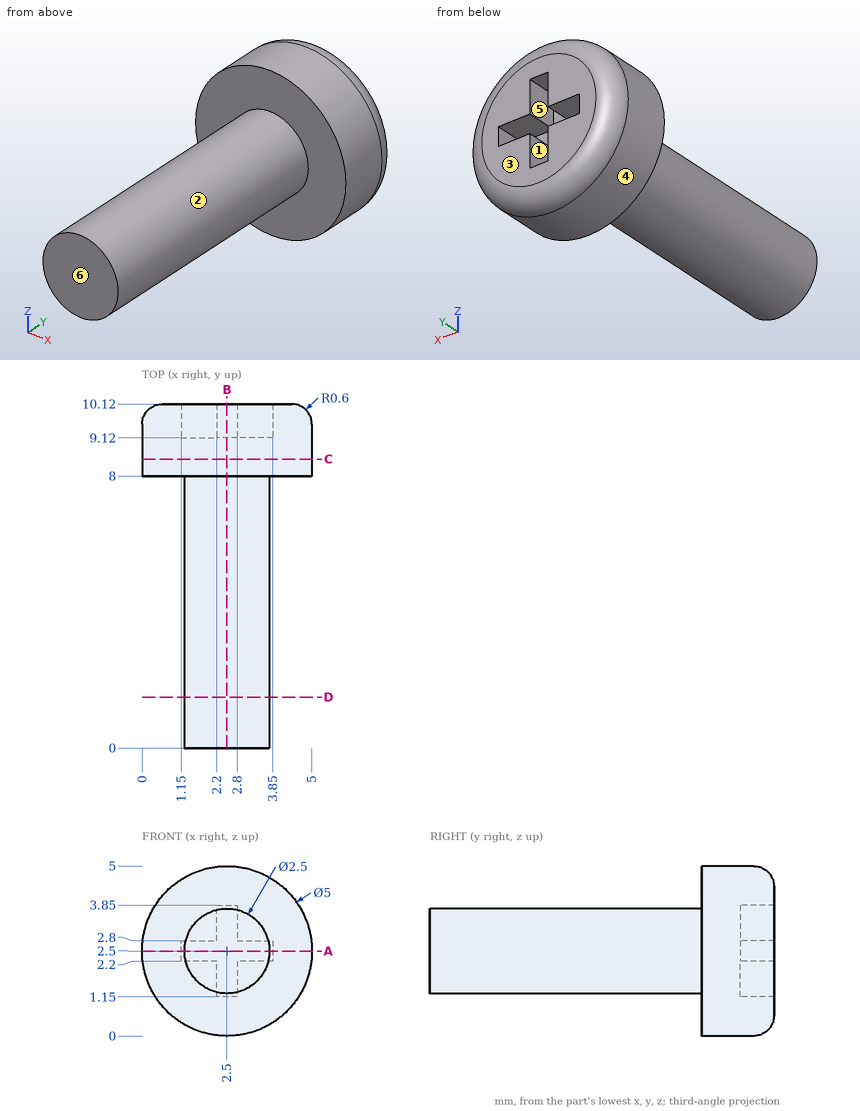
Study the drawing (mm; zero at the part's minimum x, y, z) and answer. A direction names the side the tool comes from. Coordinates: 2 decimals unless noted, no trailing zeros. Write each loop counter-clockwise with the first axis right and the second up, starting at its lowest first coordinate (ties: lowest second). Pieces come first, ordered by that corner, then holes. Notation, with made-up numbers: (-26.75, 11.25) - (-7.75, 11.25) arc R17 ccw to (-7.75, 38.25) - close; hole circle Ø6 at (-4, 67.25). An arc over 180 degrees is marked (long way). Answer as a JSON object with one key per item and string values. Group by question number.
1. Which of the six approach directions +Z, -Z, +X, -X, +Y, -Y give full straight-line access (tool end or side, diameter ignored) to the marked faces 1, 2 and 3?
2. Each of these flat-tipped pins is pushed along its axis until it touches: P1, Ø0.8, axis at x = 3.5, y = 9.5, coming from the -Z side; P2, Ø1, axis at y = 1.5, z = 0.5, coming from the -X side; P3, Ø1.5, axis at x = 3, z = 4.5, coming from the -Y side; P4, Ø1.5, axis at y = 1, z = 1, coming from the -X side. Where does it stop, or does it pass through?
3. A cutting plane is placed at C-C (y = 8.5). Determine the outline of the cut face in (x, z).
4. A cutting plane is placed at B-B (x = 2.5). Determine the outline of the cut face in (y, z), plus the area to 3 significant figures.
5. Consider L1, parallel to Y at x = 4.2, z = 2.9; L2, parallel to Y at x = 2.45, z = 2.2; L3, parallel to Z at x = 2.7, y = 8.5. Determine where each line is inside the solid, lowest interval first. Write a range as [from, to].
6. A cutting plane is placed at D-D (y = 1.5). Determine the outline of the cut face in (x, z).
7. The mould has two halves that part along X. Classify the marked faces 4, 5 and 6: +X half, -X half, draft (parallel to the pull), parting line (faces both ways), or undercut.
8. A cutting plane is placed at A-A (z = 2.5). Determine the outline of the cut face in (x, y), plus the area to 3 significant figures.
Worked out:
{
 "1": {"face 1": "+Y", "face 2": "-Y", "face 3": "+Z, -Z, +X, -X, +Y"},
 "2": {"P1": "stops at z = 0.07", "P2": "passes through", "P3": "stops at y = 8", "P4": "stops at x = 1.5"},
 "3": {"outline": "circle Ø5 at (2.5, 2.5)"},
 "4": {"outline": "(0, 1.25) - (8, 1.25) - (8, 0) - (9.52, 0) arc R0.6 ccw to (10.12, 0.6) - (10.12, 1.15) - (9.12, 1.15) - (9.12, 3.85) - (10.12, 3.85) - (10.12, 4.4) arc R0.6 ccw to (9.52, 5) - (8, 5) - (8, 3.75) - (0, 3.75) - close", "area": "27.7 mm²"},
 "5": {"L1": "y = [8, 10.12]", "L2": "y = [0, 9.12]", "L3": "z = [0.01, 4.99]"},
 "6": {"outline": "circle Ø2.5 at (2.5, 2.5)"},
 "7": {"face 4": "parting line", "face 5": "undercut", "face 6": "draft"},
 "8": {"outline": "(0, 8) - (1.25, 8) - (1.25, 0) - (3.75, 0) - (3.75, 8) - (5, 8) - (5, 9.52) arc R0.6 ccw to (4.4, 10.12) - (3.85, 10.12) - (3.85, 9.12) - (1.15, 9.12) - (1.15, 10.12) - (0.6, 10.12) arc R0.6 ccw to (0, 9.52) - close", "area": "27.7 mm²"}
}
